Verification items for the finished model (mm, model axes). Face numbers are marked on the shaded views. A direction names the side the tool comes from. Round coordinates to 2 decimals unless told otherwise and drop trailing zeros. Write each loop counter-clockwise with the first axis right and the second up, starting at its lowest first coordinate (ties: lowest second). Pieces come first, ordered by that corner, then holes.
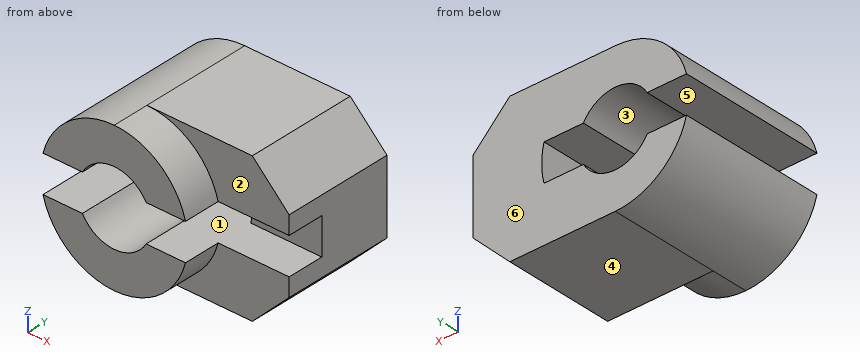
from build123d import *

# Parameters (mm, degrees)
F1_DEPTH = 20
F2_DEPTH = 15
F3_DEPTH = 10
F4_DEPTH = 25


with BuildPart() as f1:
    # F0 (on Front) → F1 (new body)
    with BuildSketch(Plane.XZ):
        with BuildLine():
            ThreePointArc((-4.330127, 2.5), (0, 5), (4.330127, 2.5))
            Line((4.330127, 2.5), (9.682458, 2.5))
            ThreePointArc((9.682458, 2.5), (6.123724, 7.905694), (0, 10))
            ThreePointArc((0, 10), (-6.123724, 7.905694), (-9.682458, 2.5))
            Line((-9.682458, 2.5), (-4.330127, 2.5))
        make_face()
        with BuildLine():
            Line((9.682458, -2.5), (4.330127, -2.5))
            ThreePointArc((4.330127, -2.5), (0, -5), (-4.330127, -2.5))
            Line((-4.330127, -2.5), (-9.682458, -2.5))
            ThreePointArc((-9.682458, -2.5), (-6.123724, -7.905694), (0, -10))
            ThreePointArc((0, -10), (6.123724, -7.905694), (9.682458, -2.5))
        make_face()
        with BuildLine():
            ThreePointArc((-5, 0), (-4.829629, 1.294095), (-4.330127, 2.5))
            Line((-4.330127, 2.5), (-9.682458, 2.5))
            ThreePointArc((-9.682458, 2.5), (-9.920297, 1.260043), (-10, 0))
            ThreePointArc((-10, 0), (-9.920297, -1.260043), (-9.682458, -2.5))
            Line((-9.682458, -2.5), (-4.330127, -2.5))
            ThreePointArc((-4.330127, -2.5), (-4.829629, -1.294095), (-5, 0))
        make_face()
    extrude(amount=F1_DEPTH)

    # F0 (on Front) → F2 (join)
    with BuildSketch(Plane.XZ):
        with BuildLine():
            ThreePointArc((0, 10), (6.123724, 7.905694), (9.682458, 2.5))
            Line((9.682458, 2.5), (19.330127, 2.5))
            Line((19.330127, 2.5), (19.330127, 5))
            Line((19.330127, 5), (14.330127, 10))
            Line((14.330127, 10), (0, 10))
        make_face()
        with BuildLine():
            Line((19.330127, -2.5), (9.682458, -2.5))
            ThreePointArc((9.682458, -2.5), (6.123724, -7.905694), (0, -10))
            Line((0, -10), (14.330127, -10))
            Line((14.330127, -10), (19.330127, -5))
            Line((19.330127, -5), (19.330127, -2.5))
        make_face()
    extrude(amount=F2_DEPTH)

    # F0 (on Front) → F3 (join)
    with BuildSketch(Plane.XZ):
        with BuildLine():
            Line((19.330127, 2.5), (9.682458, 2.5))
            ThreePointArc((9.682458, 2.5), (10, 0), (9.682458, -2.5))
            Line((9.682458, -2.5), (19.330127, -2.5))
            Line((19.330127, -2.5), (19.330127, 0))
            Line((19.330127, 0), (19.330127, 2.5))
        make_face()
    extrude(amount=F3_DEPTH)

    # F0 (on Front) → F4 (cut)
    with BuildSketch(Plane.XZ):
        with BuildLine():
            ThreePointArc((-5, 0), (-4.829629, 1.294095), (-4.330127, 2.5))
            Line((-4.330127, 2.5), (-9.682458, 2.5))
            ThreePointArc((-9.682458, 2.5), (-9.920297, 1.260043), (-10, 0))
            ThreePointArc((-10, 0), (-9.920297, -1.260043), (-9.682458, -2.5))
            Line((-9.682458, -2.5), (-4.330127, -2.5))
            ThreePointArc((-4.330127, -2.5), (-4.829629, -1.294095), (-5, 0))
        make_face()
    extrude(amount=F4_DEPTH, mode=Mode.SUBTRACT)


solid = f1.part
Q1. Release check for a two-part mould opening along Z. For the marked faces 4, 5 and 6 record: released by +Z, released by -Z, zero draft, split by the parting line, or undercut.
Recorded:
face 4: released by -Z
face 5: undercut
face 6: zero draft
Q2. Sectioned sample at C-C (x = -2). Enter the section's corners in (y, z).
Recorded:
outline: (-20, -9.8) - (0, -9.8) - (0, -4.58) - (-20, -4.58) - close; (-20, 4.58) - (0, 4.58) - (0, 9.8) - (-20, 9.8) - close
Q3. Material ranges on line 1 along Z through (x, y) = (6.25, -12); line 2 along Y through (x, z) = (12.25, 7); line 3 along Z through (x, y) = (-5, -9.25), recorded low to high.
Recorded:
line 1: z = -10 to -2.5, 2.5 to 10
line 2: y = -15 to 0
line 3: z = -8.66 to -2.5, 2.5 to 8.66
Q4. Sectioned sample at A-A (y = -17.25). Enter the section's corners in (x, z).
Recorded:
outline: (-9.68, -2.5) arc R10 ccw to (0, -10) arc R10 ccw to (9.68, -2.5) - (4.33, -2.5) arc R5 cw to (-4.33, -2.5) - close; (-9.68, 2.5) - (-4.33, 2.5) arc R5 cw to (4.33, 2.5) - (9.68, 2.5) arc R10 ccw to (0, 10) arc R10 ccw to start
Q5. Sectioned sample at B-B (x = 11.5). Enter the section's corners in (y, z), plus the area to 3 significant figures.
Recorded:
outline: (-15, -10) - (0, -10) - (0, 10) - (-15, 10) - (-15, 2.5) - (-10, 2.5) - (-10, -2.5) - (-15, -2.5) - close
area: 275 mm2
Q6. Tool access check on the marked faces 1, 2 and 3. Record the directions out of +Z, -Z, +X, -X, +Y, -Y that give a thin tool (end or side, any length) a straight path to the whole face; none if there is none.
Recorded:
face 1: -X, -Y
face 2: +Z, +X, -Y
face 3: +Y, -Y
Q7. Sectioned sample at D-D (y = -1.5). Enter the section's corners in (x, z), plus the area to 3 significant figures.
Recorded:
outline: (-9.68, -2.5) arc R10 ccw to (0, -10) - (14.33, -10) - (19.33, -5) - (19.33, 5) - (14.33, 10) - (0, 10) arc R10 ccw to (-9.68, 2.5) - (-4.33, 2.5) arc R5 cw to (4.33, 2.5) - (9.68, 2.5) arc R10 cw to (9.68, -2.5) - (4.33, -2.5) arc R5 cw to (-4.33, -2.5) - close
area: 389 mm2
Q8. Depth check by flat-ended pin: P1, Ø1, axis at y = -17.5, z = -7.5, coming from the +X side; P2, Ø2.5, axis at x = 16.5, z = 0.5, coming from the -Y side; P3, Ø4, axis at x = 13.5, z = 8, coming from the -Y side. Enter the tip coordinate at first touch or a pass-through.
Recorded:
P1: stops at x = 7.14
P2: stops at y = -10
P3: stops at y = -15
